Input: part model. Units: mm. Frame: model coordinates. A direction names the side the tool comes from. Coordinates: 2 decimals unless noted, no trailing zeros. Loops run counter-clockwise (first coordinate to the right, second up) from the corner with the lowest first, then second, coordinate; pieces in that order, holes last. Notation, with made-up numbers: (56.25, 19) - (101.25, 19) arc R18 ccw to (101.25, 24) - close; hole circle Ø1 at (1.5, -28.5). An arc over 180 degrees is marked (long way). Use a Markdown table: item, result. Add a question column.
1. Access query for faces 1 (the face through (5, 0, -2)), 2 (the face through (0, 6, 0)). Directions: +Z, -Z, +X, -X, +Y, -Y. A direction counts if a zero-diameter tool reaches every point of the face in a straight line with its end or side. Return the directions, or none.
2. Draft query along Z for faces 3 (the face through (0, 5, -6.7)), 4 (the face through (-1.02, 2.96, 4.59)), 5 (the face through (0, 10, 0)). Return one class per face: released by +Z, released by -Z, zero draft, split by the parting line, or undercut.
3. Section query C-C on z = 0. Return the cut outline in (x, y), then the cut area to 3 significant figures.
4. Ray query, L1, parallel to X at y = 1.35, z = 0; L2, parallel to Y at x = -4, z = 1.25. Return the intervals inside material, ascending. Write a range as [from, to].
5. Section query A-A on y = 3.25. Return the cut outline in (x, z).
6. Contact query for a flat-ended pin moving along its axis: P1, Ø4.5, axis at x = -1.5, z = 0.5, coming from the -Y side. Output: stop coordinate, or through.
7. Section query B-B on x = 0. Return the cut outline in (y, z), then the cut area to 3 significant figures.
```python
from build123d import *

# Parameters (mm, degrees)
SKETCH1_R           = 4.7
BOSS_EXTRUDE1_DEPTH = 6
SKETCH2_W           = 13.4
SKETCH2_H           = 13.4
BOSS_EXTRUDE2_DEPTH = 4


with BuildPart() as part:
    # Sketch1 → Boss-Extrude1 (new body)
    with BuildSketch(Plane(origin=(0, 0, 0), x_dir=(1, 0, 0), z_dir=(0, 1, 0))):
        Polygon((0, -6.7), (-6.7, -6.7), (-6.7, 6.7), (6.7, 6.7), (6.7, -6.7), align=None)
        Circle(SKETCH1_R, mode=Mode.SUBTRACT)
    extrude(amount=BOSS_EXTRUDE1_DEPTH)

    # Sketch2 → Boss-Extrude2 (add)
    with BuildSketch(Plane(origin=(0, 6, 0), x_dir=(1, 0, 0), z_dir=(0, 1, 0))):
        Rectangle(SKETCH2_W, SKETCH2_H)
    extrude(amount=BOSS_EXTRUDE2_DEPTH)


solid = part.part
```
Resolved:
| question | item | result |
|---|---|---|
| 1 | face 1 | +Z, -Z, +X, -X, -Y |
| 1 | face 2 | -Y |
| 2 | face 3 | released by -Z |
| 2 | face 4 | undercut |
| 2 | face 5 | zero draft |
| 3 | outline | (-6.7, 0) - (-4.7, 0) - (-4.7, 6) - (4.7, 6) - (4.7, 0) - (6.7, 0) - (6.7, 10) - (-6.7, 10) - close |
| 3 | area | 77.6 mm² |
| 4 | L1 | [-6.7, -4.7], [4.7, 6.7] |
| 4 | L2 | [6, 10] |
| 5 | outline | (-6.7, -6.7) - (6.7, -6.7) - (6.7, 6.7) - (-6.7, 6.7) - close; hole circle Ø9.4 at (0, 0) |
| 6 | P1 | y = 6 |
| 7 | outline | (0, -6.7) - (10, -6.7) - (10, 6.7) - (0, 6.7) - (0, 4.7) - (6, 4.7) - (6, -4.7) - (0, -4.7) - close |
| 7 | area | 77.6 mm² |
